Part model, mm, in its own coordinate system. A direction names the side the tool comes from. Give positions to 0.01 mm unless a question says otherwise; leave off trailing zeros. Order: outer loops, then holes, each group sorted by start corner. A loop starts at its lowest first (then second) coordinate and runs counter-clockwise, first axis right, second up.
1. Mould opens along X. For faces 1 (the flat face through (-1, 9, 75)), 2 (the flat face through (-125, 4, 2)), 3 (the flat face through (125, 4, 2)) say: +X half, -X half, draft (parallel to the pull), parting line (faces both ways), or undercut.
2. Slice it at B-B on z = 7.5. List the corners of the cut face in (x, y), and give its area (3 significant figures).
3. Which spindle directions (+Z, -Z, +X, -X, +Y, -Y) get a long thin tool onto all of the face, cutting with end or side? Do faces 4 (the flat face through (-2, 9, 125)), 5 (the flat face through (-1, 9, -75)). Say none if no direction does.
4. Probe line 1 (X direction, y = 2, z = -38); line 2 (X direction, y = 12.75, z = 29.5). List the from-to ranges inside material, lowest first.
5. Slice it at A-A on x = 31. List the corners of the cut face in (y, z), and give its area (3 significant figures).
6. Slice it at C-C on y = 15.25. List the corners of the cut face in (x, z).
7. Slice it at D-D on x = 69.5. List the corners of the cut face in (y, z).
from build123d import *

# Parameters (mm, degrees)
SKETCH_1_W      = 250
SKETCH_1_H      = 250
SKETCH_1_W_2    = 150
SKETCH_1_H_2    = 150
EXTRUDE_1_DEPTH = 18
FILLET_1_R      = 10
FILLET_2_R      = 10


with BuildPart() as part:
    # 草图1 → 凸台-拉伸1 (new body)
    with BuildSketch(Plane(origin=(0, 0, 0), x_dir=(1, 0, 0), z_dir=(0, 1, 0))):
        Rectangle(SKETCH_1_W, SKETCH_1_H)
        Rectangle(SKETCH_1_W_2, SKETCH_1_H_2, mode=Mode.SUBTRACT)
    extrude(amount=EXTRUDE_1_DEPTH)

    # 圆角1
    fillet_1_edges = [part.edges().sort_by_distance(p)[0] for p in [
        (125, 18, 0),
        (-125, 18, 0),
    ]]
    fillet(fillet_1_edges, radius=FILLET_1_R)

    # 圆角2
    fillet_2_edges = [part.edges().sort_by_distance(p)[0] for p in [
        (-75, 9, -75),
        (-75, 9, 75),
        (75, 9, 75),
        (75, 9, -75),
    ]]
    fillet(fillet_2_edges, radius=FILLET_2_R)


solid = part.part
Data:
1. face 1: undercut
1. face 2: -X half
1. face 3: +X half
2. outline: (-125, 0) - (-75, 0) - (-75, 18) - (-115, 18) arc R10 ccw to (-125, 8) - close; (75, 0) - (125, 0) - (125, 8) arc R10 ccw to (115, 18) - (75, 18) - close
2. area: 1,760 mm2
3. face 4: +Z, +X, -X, +Y, -Y
3. face 5: +Y, -Y
4. line 1: x = -125 to -75, 75 to 125
4. line 2: x = -123.8 to -75, 75 to 123.8
5. outline: (0, -125) - (18, -125) - (18, -75) - (0, -75) - close; (0, 75) - (18, 75) - (18, 125) - (0, 125) - close
5. area: 1,800 mm2
6. outline: (-121.89, -125) - (121.89, -125) - (121.89, 125) - (-121.89, 125) - close; hole (-75, -65) arc R10 ccw to (-65, -75) - (65, -75) arc R10 ccw to (75, -65) - (75, 65) arc R10 ccw to (65, 75) - (-65, 75) arc R10 ccw to (-75, 65) - close
7. outline: (0, -125) - (18, -125) - (18, -73.93) - (0, -73.93) - close; (0, 73.93) - (18, 73.93) - (18, 125) - (0, 125) - close
